from build123d import *

# Parameters (mm, degrees)
SKETCH1_R           = 1.5875
BOSS_EXTRUDE1_DEPTH = 0.7366


with BuildPart() as part:
    # Sketch1 → Boss-Extrude1 (new body)
    with BuildSketch(Plane.XY):
        with BuildLine():
            Line((-16.764, -26.9875), (-16.764, -31.4325))
            ThreePointArc((-16.764, -31.4325), (-16.373426893, -32.375426893), (-15.4305, -32.766))
            Line((-15.4305, -32.766), (15.4305, -32.766))
            ThreePointArc((15.4305, -32.766), (16.373426893, -32.375426893), (16.764, -31.4325))
            Line((16.764, -31.4325), (16.764, -26.9875))
            ThreePointArc((16.764, -26.9875), (17.898521883, -24.248521883), (20.6375, -23.114))
            Line((20.6375, -23.114), (22.225, -23.114))
            ThreePointArc((22.225, -23.114), (24.290458908, -22.258458908), (25.146, -20.193))
            Line((25.146, -20.193), (25.146, 20.193))
            ThreePointArc((25.146, 20.193), (24.290458908, 22.258458908), (22.225, 23.114))
            Line((22.225, 23.114), (20.6375, 23.114))
            ThreePointArc((20.6375, 23.114), (17.898521883, 24.248521883), (16.764, 26.9875))
            Line((16.764, 26.9875), (16.764, 39.0525))
            ThreePointArc((16.764, 39.0525), (15.908458908, 41.117958908), (13.843, 41.9735))
            Line((13.843, 41.9735), (-13.843, 41.9735))
            ThreePointArc((-13.843, 41.9735), (-15.908458908, 41.117958908), (-16.764, 39.0525))
            Line((-16.764, 39.0525), (-16.764, 26.9875))
            ThreePointArc((-16.764, 26.9875), (-17.898521883, 24.248521883), (-20.6375, 23.114))
            Line((-20.6375, 23.114), (-22.225, 23.114))
            ThreePointArc((-22.225, 23.114), (-24.290458908, 22.258458908), (-25.146, 20.193))
            Line((-25.146, 20.193), (-25.146, -20.193))
            ThreePointArc((-25.146, -20.193), (-24.290458908, -22.258458908), (-22.225, -23.114))
            Line((-22.225, -23.114), (-20.6375, -23.114))
            ThreePointArc((-20.6375, -23.114), (-17.898521883, -24.248521883), (-16.764, -26.9875))
        make_face()
        with Locations((-22.225, 20.193)):
            Circle(SKETCH1_R, mode=Mode.SUBTRACT)
        with Locations((22.225, 20.193)):
            Circle(SKETCH1_R, mode=Mode.SUBTRACT)
        with Locations((22.225, -20.193)):
            Circle(SKETCH1_R, mode=Mode.SUBTRACT)
        with Locations((-22.225, -20.193)):
            Circle(SKETCH1_R, mode=Mode.SUBTRACT)
        with BuildLine():
            Line((15.113, -27.305), (15.113, -18.9865))
            ThreePointArc((15.113, -18.9865), (15.503573107, -18.043573107), (16.4465, -17.653))
            Line((16.4465, -17.653), (19.685, -17.653))
            ThreePointArc((19.685, -17.653), (22.379076836, -16.537076836), (23.495, -13.843))
            Line((23.495, -13.843), (23.495, 13.843))
            ThreePointArc((23.495, 13.843), (22.379076836, 16.537076836), (19.685, 17.653))
            Line((19.685, 17.653), (16.4465, 17.653))
            ThreePointArc((16.4465, 17.653), (15.503573107, 18.043573107), (15.113, 18.9865))
            Line((15.113, 18.9865), (15.113, 36.5125))
            ThreePointArc((15.113, 36.5125), (13.997076836, 39.206576836), (11.303, 40.3225))
            Line((11.303, 40.3225), (-11.303, 40.3225))
            ThreePointArc((-11.303, 40.3225), (-13.997076836, 39.206576836), (-15.113, 36.5125))
            Line((-15.113, 36.5125), (-15.113, 18.9865))
            ThreePointArc((-15.113, 18.9865), (-15.503573107, 18.043573107), (-16.4465, 17.653))
            Line((-16.4465, 17.653), (-19.685, 17.653))
            ThreePointArc((-19.685, 17.653), (-22.379076836, 16.537076836), (-23.495, 13.843))
            Line((-23.495, 13.843), (-23.495, -13.843))
            ThreePointArc((-23.495, -13.843), (-22.379076836, -16.537076836), (-19.685, -17.653))
            Line((-19.685, -17.653), (-16.4465, -17.653))
            ThreePointArc((-16.4465, -17.653), (-15.503573107, -18.043573107), (-15.113, -18.9865))
            Line((-15.113, -18.9865), (-15.113, -27.305))
            ThreePointArc((-15.113, -27.305), (-13.997076836, -29.999076836), (-11.303, -31.115))
            Line((-11.303, -31.115), (11.303, -31.115))
            ThreePointArc((11.303, -31.115), (13.997076836, -29.999076836), (15.113, -27.305))
        make_face(mode=Mode.SUBTRACT)
    extrude(amount=BOSS_EXTRUDE1_DEPTH)


solid = part.part
Source: CAD feature listing. Evaluate the final solid. Frame: model axes, mm. A direction names the side the tool comes from. Round coordinates to 2 decimals unless told otherwise and drop trailing zeros. Order: outer loops, then holes, each group sorted by start corner. A loop starts at its lowest first (then second) coordinate and runs counter-clockwise, first axis right, second up. Notation, with made-up numbers: (31.25, 69.5) -> (60.25, 69.5) arc R30 cw to (60.25, 99.5) -> close; hole circle Ø1 at (29.5, -13). An arc over 180 degrees is marked (long way). Answer as CSV lines item,"result".
Item 1: Reachability of faces 5 (the face through (-22.349, 16.567, 0.363)), 6 (the face through (17.93, 24.22, 0.36)) from +Z, -Z, +X, -X, +Y, -Y: full face, straight path, thin tool, end or side. Return the list, or none.
A:
face 5,"+Z, -Z"
face 6,"+Z, -Z, +X, +Y"
Item 2: Section A-A, the plane y = -3. Return loops of the section in (x, z) (3 decimals), plus the area to 3 significant figures.
A:
outline,"(-25.146, 0) -> (-23.495, 0) -> (-23.495, 0.737) -> (-25.146, 0.737) -> close; (23.495, 0) -> (25.146, 0) -> (25.146, 0.737) -> (23.495, 0.737) -> close"
area,"2.43 mm²"
Item 3: Section B-B, the plane x = -7. Return loops of the section in (y, z) (1 decimal).
A:
outline,"(-32.8, 0) -> (-31.1, 0) -> (-31.1, 0.7) -> (-32.8, 0.7) -> close; (40.3, 0) -> (42, 0) -> (42, 0.7) -> (40.3, 0.7) -> close"
Item 4: Pull-direction query (X, two-part tool) for faces 1 (the face through (22.409, 16.507, 0.363)), 2 (the face through (17.87, -24.28, 0.36)), 3 (the face through (-20.76, -20.8, 0.36)), 4 (the face through (-24.31, -22.24, 0.36)); classes: pulls with the +X half, pulls with the -X half, needs draft (parallel to the pull), parting line crosses it, or undercut.
A:
face 1,"undercut"
face 2,"pulls with the +X half"
face 3,"undercut"
face 4,"pulls with the -X half"
Item 5: Section C-C, the plane z = 0.5. Count the separate pieces of the cut face and the enclosed holes in it, plus the area to 3 significant figures.
A:
separate pieces,"1"
enclosed holes,"5"
area,"523 mm²"
Item 6: Line query: L1, parallel to X at y = 14, z = 0.4; L2, parallel to Y at x = 0, z = 0.55 (1 decimal); L3, parallel to X at y = 35, z = 0.35. Output: solid intervals per line, ascending.
A:
L1,"-25.15 to -23.49, 23.49 to 25.15"
L2,"-32.8 to -31.1, 40.3 to 42"
L3,"-16.76 to -15.11, 15.11 to 16.76"
